Input: part model. Units: mm. Frame: model coordinates. Give positions to 0.01 mm unless a question says otherwise; leave off trailing zeros. Loops run counter-clockwise (first coordinate to the right, second up) from the corner with the lowest first, then second, coordinate; pieces in that order, holes last. Notation, with made-up numbers: (75, 53) - (128, 53) arc R30 ccw to (128, 85) - close; hole circle Ø5 at (81, 79). An arc over 180 degrees is marked (long way). One line per question, with ' | ' between items. Start each with the question number.
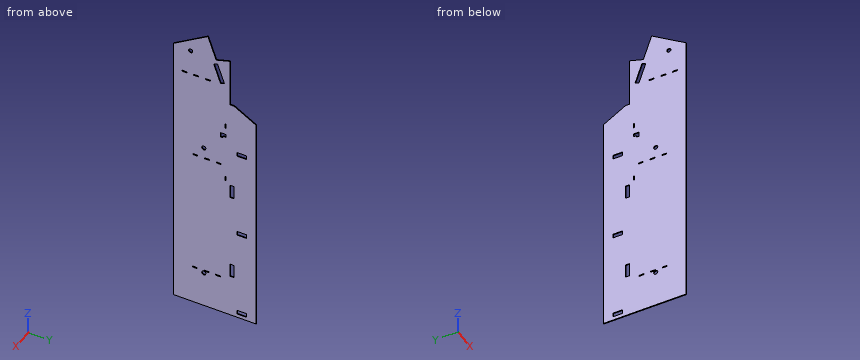
from build123d import *

# Parameters (mm, degrees)
SKETCH1_W           = 4
SKETCH1_H           = 17
SKETCH1_W_2         = 17
SKETCH1_H_2         = 4
SKETCH1_W_3         = 14.5201
SKETCH1_H_3         = 33.8773
SKETCH1_W_4         = 48.399
SKETCH1_H_4         = 14.5267
SKETCH1_W_5         = 48.409
SKETCH1_H_5         = 14.5201
SKETCH1_H_6         = 16.9197
SKETCH1_H_7         = 16.9198
BOSS_EXTRUDE2_DEPTH = 3


with BuildPart() as part:
    # Sketch1 → Boss-Extrude2 (new body)
    with BuildSketch(Plane(origin=(0, 0, 0), x_dir=(0, 0, -1), z_dir=(1, 0, 0))):
        Polygon((-503.9458, -26.8502), (-427.6871, -148.1709), (573.7687, -148.1709), (573.7687, 142.5497), (-218.3839, 142.5497), (-263.2513, 65.0539), (-263.2513, 50.6289), (-436.1861, 50.5939), (-421.6644, 2.1883), align=None)
        with Locations((434.7463, 9.1594)):
            Rectangle(SKETCH1_W, SKETCH1_H, mode=Mode.SUBTRACT)
        with Locations((37.2084, 34.4461)):
            Rectangle(SKETCH1_W_2, SKETCH1_H_2, mode=Mode.SUBTRACT)
        Polygon((-408.1165, 7.0272), (-339.6566, 31.1916), (-334.8227, 17.4953), (-403.2826, -6.6625), align=None, mode=Mode.SUBTRACT)
        with Locations((-75.60135, 91.73875)):
            Rectangle(SKETCH1_W_3, SKETCH1_H_3, mode=Mode.SUBTRACT)
        with Locations((81.6996, 57.85395)):
            Rectangle(SKETCH1_W_4, SKETCH1_H_4, mode=Mode.SUBTRACT)
        with Locations((239.00055, 91.73875)):
            Rectangle(SKETCH1_W_3, SKETCH1_H_3, mode=Mode.SUBTRACT)
        with Locations((396.3082, 57.85895)):
            Rectangle(SKETCH1_W_5, SKETCH1_H_5, mode=Mode.SUBTRACT)
        with Locations((553.60245, 91.73875)):
            Rectangle(SKETCH1_W_3, SKETCH1_H_3, mode=Mode.SUBTRACT)
        with Locations((-331.1886, -27.0339)):
            Rectangle(SKETCH1_W, SKETCH1_H, mode=Mode.SUBTRACT)
        with Locations((-331.1886, -68.18055)):
            Rectangle(SKETCH1_W, SKETCH1_H_6, mode=Mode.SUBTRACT)
        with Locations((-331.1886, -109.3272)):
            Rectangle(SKETCH1_W, SKETCH1_H, mode=Mode.SUBTRACT)
        with Locations((-171.5395, 34.4461)):
            Rectangle(SKETCH1_W_2, SKETCH1_H_2, mode=Mode.SUBTRACT)
        Polygon((-127.6656, 36.4461), (-127.6656, 26.4461), (-121.933, 26.4461), (-121.933, 17.3384), (-138.8528, 17.3384), (-138.8528, 36.4461), align=None, mode=Mode.SUBTRACT)
        with Locations((-14, 11.2)):
            Rectangle(SKETCH1_W, SKETCH1_H, mode=Mode.SUBTRACT)
        with Locations((-14, -29.9466)):
            Rectangle(SKETCH1_W, SKETCH1_H_7, mode=Mode.SUBTRACT)
        with Locations((-14, -71.0932)):
            Rectangle(SKETCH1_W, SKETCH1_H, mode=Mode.SUBTRACT)
        with Locations((434.7463, -31.9872)):
            Rectangle(SKETCH1_W, SKETCH1_H_7, mode=Mode.SUBTRACT)
        with Locations((434.7463, -73.1338)):
            Rectangle(SKETCH1_W, SKETCH1_H, mode=Mode.SUBTRACT)
        with BuildLine():
            add(Edge.make_bspline(
                [(444.7022, -48.6335), (440.6903, -48.6335), (437.4421, -45.382), (437.4421, -41.3735)],
                knots=[0, 0, 0, 0, 0.333333333, 0.333333333, 0.333333333, 0.333333333], degree=3))
            add(Edge.make_bspline(
                [(437.4421, -41.3735), (437.4421, -37.3617), (440.6937, -34.1135), (444.7022, -34.1135)],
                knots=[0.333333333, 0.333333333, 0.333333333, 0.333333333, 1, 1, 1, 1], degree=3))
            add(Edge.make_bspline(
                [(444.7022, -34.1135), (448.7124, -34.1135), (451.9639, -37.3617), (451.9639, -41.3735)],
                knots=[0, 0, 0, 0, 0.333333333, 0.333333333, 0.333333333, 0.333333333], degree=3))
            add(Edge.make_bspline(
                [(451.9639, -41.3735), (451.9639, -45.372), (448.7124, -48.6335), (444.7022, -48.6335)],
                knots=[0.333333333, 0.333333333, 0.333333333, 0.333333333, 1, 1, 1, 1], degree=3))
        make_face(mode=Mode.SUBTRACT)
        with BuildLine():
            add(Edge.make_bspline(
                [(-53.8196, -48.6335), (-57.8298, -48.6335), (-61.0797, -45.382), (-61.0797, -41.3735)],
                knots=[0, 0, 0, 0, 0.333333333, 0.333333333, 0.333333333, 0.333333333], degree=3))
            add(Edge.make_bspline(
                [(-61.0797, -41.3735), (-61.0797, -37.3617), (-57.8282, -34.1135), (-53.8196, -34.1135)],
                knots=[0.333333333, 0.333333333, 0.333333333, 0.333333333, 1, 1, 1, 1], degree=3))
            add(Edge.make_bspline(
                [(-53.8196, -34.1135), (-49.8111, -34.1135), (-46.5596, -37.3617), (-46.5596, -41.3735)],
                knots=[0, 0, 0, 0, 0.333333333, 0.333333333, 0.333333333, 0.333333333], degree=3))
            add(Edge.make_bspline(
                [(-46.5596, -41.3735), (-46.5596, -45.372), (-49.8111, -48.6335), (-53.8196, -48.6335)],
                knots=[0.333333333, 0.333333333, 0.333333333, 0.333333333, 1, 1, 1, 1], degree=3))
        make_face(mode=Mode.SUBTRACT)
        with BuildLine():
            add(Edge.make_bspline(
                [(-422.3548, -94.6631), (-426.3633, -94.6631), (-429.6148, -91.4116), (-429.6148, -87.4031)],
                knots=[0, 0, 0, 0, 0.333333333, 0.333333333, 0.333333333, 0.333333333], degree=3))
            add(Edge.make_bspline(
                [(-429.6148, -87.4031), (-429.6148, -83.3946), (-426.3633, -80.1431), (-422.3548, -80.1431)],
                knots=[0.333333333, 0.333333333, 0.333333333, 0.333333333, 1, 1, 1, 1], degree=3))
            add(Edge.make_bspline(
                [(-422.3548, -80.1431), (-418.3462, -80.1431), (-415.0947, -83.3946), (-415.0947, -87.4031)],
                knots=[0, 0, 0, 0, 0.333333333, 0.333333333, 0.333333333, 0.333333333], degree=3))
            add(Edge.make_bspline(
                [(-415.0947, -87.4031), (-415.0947, -91.4116), (-418.3462, -94.6631), (-422.3548, -94.6631)],
                knots=[0.333333333, 0.333333333, 0.333333333, 0.333333333, 1, 1, 1, 1], degree=3))
        make_face(mode=Mode.SUBTRACT)
    extrude(amount=BOSS_EXTRUDE2_DEPTH)


solid = part.part
Q1. First-contact query: pin 1 (0.9 mm diameter, centred on x = 2, y = 100, fed in from +Z); pin 2 (1.5 mm diameter, centred on x = 1.5, y = 34.5, fed in from +Z); pin 3 (1.5 mm diameter, centred on x = 2, y = -29.5, fed in from +Z). Flat tips, straight axial feed; report the tip coordinate or a pass-through.
Q2. Line query: L1, parallel to Y at x = 1.3, z = -235; L2, parallel to Y at x = 1.55, z = -34.5; L3, parallel to Y at x = 0.45, z = 327. Output: solid intervals per line, ascending. Write a range as from..to.
Q3. Section B-B, the plane x = 2.5. Count the separate pieces of the cut face and the enclosed holes in it, plus the area to 3 significant figures.
Q4. Section A-A, the plane y = -129.5. Output: boundary loops of the cut face in (x, z), plus the area to 3 significant figures.
Solved:
1) pin 1: stops at z = 243.28 | pin 2: stops at z = 431.58 | pin 3: stops at z = 502.75
2) L1: y = -148.17..74.8, 108.68..142.55 | L2: y = -148.17..32.45, 36.45..142.55 | L3: y = -148.17..50.62
3) separate pieces: 1 | enclosed holes: 21 | area: 275,000 mm²
4) outline: (0, -573.77) - (3, -573.77) - (3, 439.42) - (0, 439.42) - close | area: 3,040 mm²
